Part model, mm, in its own coordinate system. Face numbers are marked on the shaded views. A direction names the side the tool comes from. Give positions to 0.01 mm unless a question says otherwise; leave off trailing zeros. Order: outer loops, then holes, each group sorted by start corner. A loop starts at its lowest first (then second) coordinate and runs counter-clockwise, first axis right, second up. Notation, with made-up numbers: M 71,20.25 L 91,20.25 A32 cw 91,54.25 Z; hole C 23,9.5 d8. An arc over 180 degrees is marked long. Answer as a JSON object with one key per item and string values.
from build123d import *

# Parameters (mm, degrees)
F0_R     = 68.2587577657
F1_DEPTH = 10
F2_R     = 60.1472105794
F3_DEPTH = 5
F4_R     = 56.5410055919
F5_DEPTH = 7
F6_T     = 10


with BuildPart() as f1:
    # F0 (on Top) → F1 (new body)
    with BuildSketch(Plane.XY):
        Circle(F0_R)
    extrude(amount=F1_DEPTH)

    # F2 (on face) → F3 (join)
    with BuildSketch(Plane.XY.offset(10)):
        Circle(F2_R)
    extrude(amount=-F3_DEPTH)

    # F4 (on face) → F5 (join)
    with BuildSketch(Plane.XY.offset(10)):
        Circle(F4_R)
    extrude(amount=-F5_DEPTH)

    # F6
    f6_openings = [f1.faces().sort_by_distance(p)[0] for p in [
        (0, 0, 10),
    ]]
    offset(amount=F6_T, openings=f6_openings, kind=Kind.INTERSECTION)


solid = f1.part
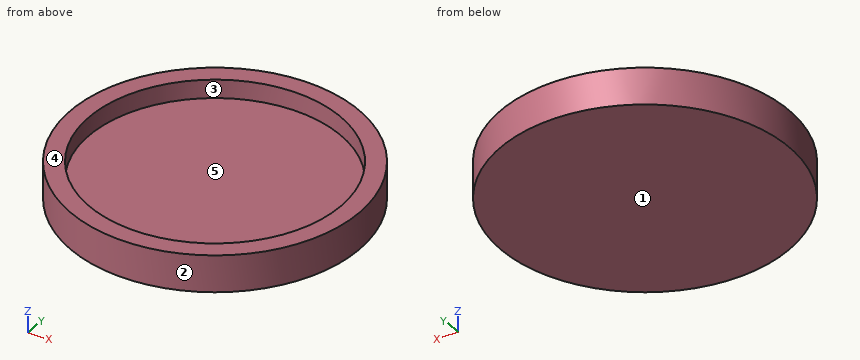
1. Cut at C-C on z = 5. Give the cut face in (x, y), plus the area to 3 significant figures.
Worked answers:
{"outline": "C 0,0 d156.52; hole C 0,0 d136.52", "area": "4,600 mm^2"}
2. Pin check, flat tips, straight feed: P1, Ø8, axis at x = 41.5, y = 13, coming from the +Z side; P2, Ø5, axis at y = 10, z = 0, coming from the -X side; P3, Ø10, axis at x = -6.5, z = -2.5, coming from the +Y side. Stop position of each tip, or through.
Worked answers:
{"P1": "stops at z = 0", "P2": "stops at x = -77.9", "P3": "stops at y = 78.24"}
3. Cut at D-D on z = -7. Give the cut face in (x, y).
Worked answers:
{"outline": "C 0,0 d156.52"}
4. Cut at A-A on y = 0. Give the cut face in (x, z), plus the area to 3 significant figures.
Worked answers:
{"outline": "M -78.26,-10 L 78.26,-10 L 78.26,10 L 68.26,10 L 68.26,0 L -68.26,0 L -68.26,10 L -78.26,10 Z", "area": "1,770 mm^2"}
5. Which spindle directions (+Z, -Z, +X, -X, +Y, -Y) get a long thin tool onto all of the face, cutting with end or side? Do the marked faces 4 and 5. Say none if no direction does.
Worked answers:
{"face 4": "+Z, +X, -X, +Y, -Y", "face 5": "+Z"}
6. Probe line 1 along Y through (x, z) = (0, 6.5); line 2 along Z through (x, y) = (30, 33.5); line 3 along X through (y, z) = (-53.5, 4.75). List the from-to ranges inside material, lowest first.
Worked answers:
{"line 1": "y = -78.26 to -68.26, 68.26 to 78.26", "line 2": "z = -10 to 0", "line 3": "x = -57.12 to -42.39, 42.39 to 57.12"}
7. Two-plate mould, pull along X, no slides. Class the marked faces 1, 2 and 3: +X half, -X half, draft (parallel to the pull), parting line (faces both ways), or undercut.
Worked answers:
{"face 1": "draft", "face 2": "parting line", "face 3": "undercut"}
